Geometry: final body of the model. Coordinates: model frame, mm. A direction names the side the tool comes from. Round coordinates to 2 decimals unless told otherwise and drop trailing zeros. Order: outer loops, then holes, each group sorted by start corner. A loop starts at its lowest first (then second) coordinate and runs counter-clockwise, first axis right, second up. Notation, with made-up numbers: (67.25, 29.5) -> (71.25, 29.5) arc R17 cw to (71.25, 60.5) -> close; hole circle Ø8 at (85.25, -24.5). An arc over 180 degrees is marked (long way). Put each result on its own line as item: value.
Autodesk Inventor part; units mm, degrees
ref_plane "YZ Plane" through (0, 0, 0) normal (1, 0, 0) x (0, 1, 0)
ref_plane "XZ Plane" through (0, 0, 0) normal (0, 1, 0) x (-1, 0, 0)
ref_plane "XY Plane" through (0, 0, 0) normal (0, 0, 1) x (1, 0, 0)
sketch "Sketch1" plane through (0, 0, 0) normal (0, 0, 1) x (1, 0, 0)
  line L0 (279.4704, -19.05) -> (-282.4704, -19.05)
  line L1 (-282.4704, -19.05) -> (-282.4704, 19.05)
  line L2 (-282.4704, 19.05) -> (279.4704, 19.05)
  line L3 (282.4704, -19.05) -> (-282.4704, 19.05) construction
  line L4 (-282.4704, -19.05) -> (282.4704, 19.05) construction
  line L5 (292.1704, -25.05) -> (285.4704, -25.05)
  line L6 (285.4704, 25.05) -> (292.1704, 25.05)
  line L7 (295.1704, 22.05) -> (295.1704, -22.05)
  line L8 (295.1704, -25.05) -> (282.4704, 25.05) construction
  line L9 (282.4704, -25.05) -> (295.1704, 25.05) construction
  line L10 (282.4704, -22.05) -> (282.4704, -22.05)
  line L11 (282.4704, 22.05) -> (282.4704, 22.05)
  arc A0 (279.4704, 19.05) -> (282.4704, 22.05) centre (279.4704, 22.05) ccw
  arc A1 (285.4704, 25.05) -> (282.4704, 22.05) centre (285.4704, 22.05) ccw
  arc A2 (295.1704, 22.05) -> (292.1704, 25.05) centre (292.1704, 22.05) ccw
  arc A3 (292.1704, -25.05) -> (295.1704, -22.05) centre (292.1704, -22.05) ccw
  arc A4 (282.4704, -22.05) -> (285.4704, -25.05) centre (285.4704, -22.05) ccw
  arc A5 (282.4704, -22.05) -> (279.4704, -19.05) centre (279.4704, -22.05) ccw
  point P0 (0, 0)
  point P1 (288.8204, 0)
  point P2 (282.4704, 0)
  point P3 (295.1704, 0)
  dimension "d0" = 12.7
  dimension "d1" = 577.6407
  dimension "d2" = 6
  dimension "d3" = 38.1
  dimension "d4" = 3
extrude "Plate1" add sketch "Sketch1" along normal blind 4.7625
sketch "Sketch2" plane through (0, 0, 0) normal (0, 0, -1) x (-1, 0, 0)
  line L0 (-288.8204, -19.05) -> (-288.8204, 19.05)
  line L1 (-295.1704, -22.05) -> (-295.1704, 22.05)
  line L2 (-288.8204, 0) -> (-295.1704, 0)
  point P0 (0, 0)
  dimension "d6" = 6.35
  dimension "d7" = 38.1
hole "Hole1" at (288.8204, -19.05, 0) at (288.8204, 0, 0) at (288.8204, 19.05, 0) direction (0, 0, 1) diameter 5.1054 depth 4.7625 tip angle 118
sketch "Sketch3" plane through (0, 0, 0) normal (0, 0, -1) x (-1, 0, 0)
  line L0 (268.0066, 101.0778) -> (282.4704, 19.05)
  line L1 (180.2314, 85.6006) -> (268.0066, 101.0778)
  arc A0 (180.2314, 85.6006) -> (176.9524, 83.8547) centre (181.2732, 79.6918) ccw
  arc A1 (176.9524, 83.8547) -> (183.5568, 37.0593) centre (198.5568, 63.04) ccw
  line L2 (-279.4704, 19.05) -> (282.4704, 19.05)
  line L3 (282.4704, 19.05) -> (214.7497, 19.05)
  line L4 (282.4704, 19.05) -> (282.4704, -19.05)
  arc A2 (196.0756, 19.05) -> (196.0756, 31.05) centre (196.0756, 25.05) ccw
  line L5 (196.0756, 31.05) -> (193.9651, 31.05)
  line L6 (193.9651, 31.05) -> (183.5568, 37.0593)
  arc A3 (169.2665, 76.5071) -> (165.9875, 74.7612) centre (170.3084, 70.5983) ccw
  line L7 (169.8961, 54.1762) -> (13.9062, 54.1762)
  arc A4 (15.2621, 98.6253) -> (1.9766, 66.1058) centre (15.447, 79.5762) ccw
  line L8 (268.0066, 101.0778) -> (15.2621, 98.6253)
  line L9 (13.9062, 54.1762) -> (1.9766, 66.1058)
  circle A5 centre (15.447, 79.5762) radius 7.9502
  line L10 (282.4704, 19.05) -> (-279.4704, 19.05)
  point P0 (0, 0)
  point P1 (187.5919, 53.9466)
  dimension "d16" = 43.99
  dimension "d17" = 80
  dimension "d18" = 83.9136
  dimension "d19" = 30
  dimension "d20" = 6
  dimension "d21" = 83.2932
  dimension "d28" = 12
  dimension "d29" = 86.3948
  dimension "d30" = 30
  dimension "d44" = 6
  dimension "d45" = 25.4
  dimension "d46" = 38.1
  dimension "d47" = 135
  dimension "d48" = 15.9004
  dimension "d49" = 35.1262
  dimension "d50" = 252.4564
sheet face with bend "Face2" sketch "Sketch3" thickness 4.7625 toward (0, 0, 1) bend radius 4.7625
bend "Bend1"
fillet "Corner Round1" radius 6.35 5 edges at (-282.4704, 19.05, 2.3813) (-282.4704, -19.05, 2.3813) (-193.9651, 31.05, 2.3813) (-13.9062, 54.1762, 2.3813) (-169.8961, 54.1762, 2.3813)
sketch "Sketch4" plane through (0, 0, 0) normal (0, 0, -1) x (-1, 0, 0)
  line L0 (282.3739, 19.5971) -> (268.0066, 101.0778)
  arc A0 (169.8961, 54.1762) -> (183.5568, 37.0593) centre (198.5568, 63.04) ccw
  circle A1 centre (198.5568, 63.04) radius 25.4
  line L1 (177.7503, 77.6089) -> (213.1256, 83.8465)
  line L2 (213.1256, 83.8465) -> (183.9879, 42.2336)
  line L3 (183.9879, 42.2336) -> (219.3632, 48.4712)
  line L4 (173.5426, 58.6294) -> (223.5709, 67.4507)
  line L5 (282.3739, 19.5971) -> (268.0066, 101.0778)
  line L6 (262.1156, 61.3512) -> (265.4236, 42.5907)
  line L7 (196.0756, 19.05) -> (-279.4704, 19.05)
  line L8 (268.0066, 101.0778) -> (15.2621, 98.6253)
  line L9 (16.5365, 54.1762) -> (165.5437, 54.1762)
  circle A2 centre (15.447, 79.5762) radius 7.9502
  point P0 (0, 0)
  point P1 (257.7049, 86.3654)
  point P2 (272.0396, 5.0695)
  point P3 (208.4539, 0)
  point P4 (182.662, 0)
  point P5 (142.447, 77.1409)
  point P6 (91.647, 77.1409)
  dimension "d31" = 25.4
  dimension "d33" = 12.7
  dimension "d34" = 12.7
  dimension "d42" = 50.8
  dimension "d43" = 45
  dimension "d51" = 5.2605
  dimension "d52" = 19.05
  dimension "d53" = 38.1
  dimension "d54" = 19.05
  dimension "d55" = 19.05
  dimension "d56" = 76.2
  dimension "d57" = 101.6
  dimension "d58" = 22.2246
  dimension "d60" = 44.4491
  dimension "d61" = 50.8
  dimension "d62" = 76.2
hole "Hole2" at (-257.7049, 86.3654, 0) at (-262.1156, 61.3512, 0) at (-177.7503, 77.6089, 0) at (-173.5426, 58.6294, 0) at (-183.9879, 42.2336, 0) at (-219.3632, 48.4712, 0) at (-223.5709, 67.4507, 0) at (-213.1256, 83.8465, 0) at (-272.0396, 5.0695, 0) at (-265.4236, 42.5907, 0) at (-208.4539, 0, 0) at (-182.662, 0, 0) at (-142.447, 77.1409, 0) at (-91.647, 77.1409, 0) direction (0, 0, 1) diameter 5.105 end through all
equation "\"d13\" = Thickness"
equation "\"d34\" = d32"
equation "\"d40\" = Thickness"
equation "\"d5\" = Thickness"
equation "\"d22\" = BendRadius"
equation "\"d23\" = BendReliefWidth"
equation "\"d25\" = MinimumRemnant"
equation "\"d24\" = BendReliefDepth"
equation "\"d26\" = TransitionRadius"
equation "\"BendRadius\" = Thickness"
equation "\"BendReliefWidth\" = Thickness"
equation "\"BendReliefDepth\" = 0.5 * Thickness"
equation "\"CornerReliefSize\" = 4 * Thickness"
equation "\"MinimumRemnant\" = 2 * Thickness"
equation "\"TransitionRadius\" = BendRadius"
equation "\"JacobiRadiusSize\" = BendRadius"
equation "\"GapSize\" = Thickness"
properties part number "RACK_GUIDES" material "Polycarbonate, PC 1000, Clear"
1. Set-up query: faces 5 (the face through (-176.306, 42.918, 2.348)), 6 (the face through (-62, 11, 4.762)). Return all of +Z, -Z, +X, -X, +Y, -Y with unobstructed straight access to the full face (end or side cutting, diameter ignored); none if empty.
Ans:
face 5: +Z, -Z, +X
face 6: +Z, +X, -X, +Y, -Y
2. Draft query along X for faces 1 (the face through (-7.08, 61, 2.35)), 2 (the face through (-275.09, 60.91, 2.35)), 3 (the face through (-13.724, 71.815, 2.348)), 4 (the face through (-62, 11, 0)). Return one class per face: +X half, -X half, draft (parallel to the pull), parting line (faces both ways), or undercut.
Ans:
face 1: +X half
face 2: -X half
face 3: undercut
face 4: draft
3. Contact query for flat-ended pins moving along their axis: P1, Ø6.5, axis at x = 288.82, y = 19.05, coming from the +Z side; P2, Ø1.4, axis at x = -71.5, z = 1.5, coming from the -Y side. Output: stop coordinate, or through.
Ans:
P1: z = 4.76
P2: y = -19.05
4. Cut plane B-B on z = 3.65. State how many separate pieces and enclosed holes the cut face has, and give its area (3 significant figures).
Ans:
separate pieces: 1
enclosed holes: 18
area: 37,200 mm²
5. Material intervals for probe 1 along Y at (x, z) = (-90, 0.25); probe 2 along X at (y, z) = (79, 3.2); probe 3 along X at (y, z) = (60.5, 1.85), sorted ascending.
Ans:
probe 1: -19.05 to 19.05, 54.18 to 75.19, 79.09 to 99.35
probe 2: -271.9 to -179.89, -175.61 to -144.2, -140.7 to -93.4, -89.9 to -23.38, -7.52 to 3.59
probe 3: -275.16 to -264.52, -259.71 to -175.28, -171.81 to -7.58
6. Cut plane A-A on x = 73. Return loops of the section in (y, z), and give its area (3 significant figures).
Ans:
outline: (-19.05, 0) -> (19.05, 0) -> (19.05, 4.76) -> (-19.05, 4.76) -> close
area: 181 mm²
